from build123d import *

# Parameters (mm, degrees)
CUT_EXTRUDE1_DEPTH = 30
SKETCH3_R          = 10
CUT_EXTRUDE2_DEPTH = 30
CUT_EXTRUDE3_DEPTH = 31.3


with BuildPart() as part:
    # Sketch1 → Revolve1 (revolve)
    with BuildSketch(Plane(origin=(0, 0, 0), x_dir=(0, 0, -1), z_dir=(1, 0, 0)), mode=Mode.PRIVATE) as revolve1_sk:
        with BuildLine():
            Line((0, 20.5), (0, 15.75))
            Line((0, 15.75), (9.09326674, 0))
            Line((9.09326674, 0), (66.830344885, 0))
            Line((66.830344885, 0), (77.8, 19))
            Line((77.8, 19), (77.8, 23))
            Line((77.8, 23), (67.8, 23))
            ThreePointArc((67.8, 23), (64.1, 21.2), (60.4, 23))
            Line((60.4, 23), (38.5, 23))
            Line((38.5, 23), (36, 20.5))
            Line((36, 20.5), (0, 20.5))
        make_face()
    revolve(revolve1_sk.sketch.rotate(Axis((0, 0, 0), (0, 0, 1)), 90), axis=Axis((0, 0, 0), (0, 0, 1)))

    # Sketch2 → Cut-Extrude1 (cut)
    with BuildSketch(Plane.XY):
        with BuildLine():
            Line((-10.66, 8.821522369), (-10.66, -8.821522369))
            ThreePointArc((-10.66, -8.821522369), (-10.66, -10.66), (-8.821522369, -10.66))
            Line((-8.821522369, -10.66), (8.821522369, -10.66))
            ThreePointArc((8.821522369, -10.66), (10.66, -10.66), (10.66, -8.821522369))
            Line((10.66, -8.821522369), (10.66, 8.821522369))
            ThreePointArc((10.66, 8.821522369), (10.66, 10.66), (8.821522369, 10.66))
            Line((8.821522369, 10.66), (-8.821522369, 10.66))
            ThreePointArc((-8.821522369, 10.66), (-10.66, 10.66), (-10.66, 8.821522369))
        make_face()
    extrude(amount=-CUT_EXTRUDE1_DEPTH, mode=Mode.SUBTRACT)

    # Sketch3 → Cut-Extrude2 (cut)
    with BuildSketch(Plane.XY.offset(-30)):
        Circle(SKETCH3_R)
    extrude(amount=-CUT_EXTRUDE2_DEPTH, mode=Mode.SUBTRACT)

    # Sketch4 → Cut-Extrude3 (cut)
    with BuildSketch(Plane(origin=(0, 0, -77.8), x_dir=(-1, 0, 0), z_dir=(0, 0, -1))):
        with BuildLine():
            Line((-12.85, -9.668019485), (-12.85, 9.668019485))
            ThreePointArc((-12.85, 9.668019485), (-12.85, 12.85), (-9.668019485, 12.85))
            Line((-9.668019485, 12.85), (9.668019485, 12.85))
            ThreePointArc((9.668019485, 12.85), (12.85, 12.85), (12.85, 9.668019485))
            Line((12.85, 9.668019485), (12.85, -9.668019485))
            ThreePointArc((12.85, -9.668019485), (12.85, -12.85), (9.668019485, -12.85))
            Line((9.668019485, -12.85), (-9.668019485, -12.85))
            ThreePointArc((-9.668019485, -12.85), (-12.85, -12.85), (-12.85, -9.668019485))
        make_face()
    extrude(amount=-CUT_EXTRUDE3_DEPTH, mode=Mode.SUBTRACT)


solid = part.part
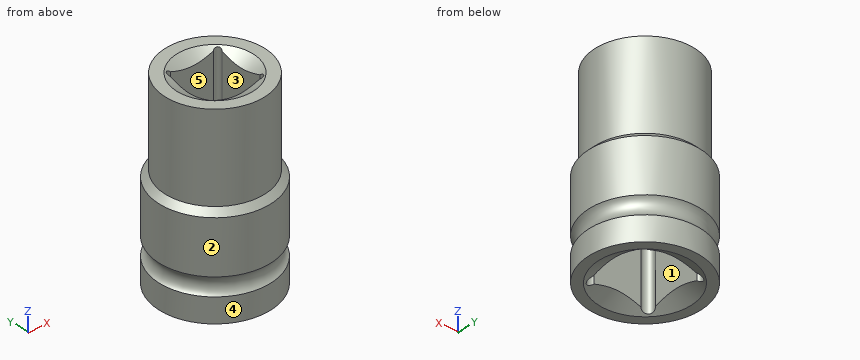
Source: CAD feature listing. Evaluate the final solid. Frame: model axes, mm. Face numbers are marked on the shaded views. A direction names the side the tool comes from. Give positions to 0.01 mm unless a question says otherwise; leave off trailing zeros. Write each loop counter-clockwise with the first axis right and the second up, starting at its lowest first coordinate (ties: lowest second). Pieces come first, ordered by that corner, then holes. Notation, with made-up numbers: M -28.75,-17 L -20.75,-17 A10 cw -20.75,2 Z; hole C -33,-15.75 d11. An arc over 180 degrees is marked long. Answer as a JSON object with one key per item and string values.
Q1. Ray query, line 1 along Y through (x, z) = (0, -41); line 2 along Y through (x, z) = (0, -35); line 3 along X through (y, z) = (-13, -50). Return the intervals inside material, ascending.
Geometry check:
{"line 1": "y = -23 to -10, 10 to 23", "line 2": "y = -20.5 to -10, 10 to 20.5", "line 3": "x = -18.97 to -12.68, -9.83 to 9.83, 12.68 to 18.97"}
Q2. Mould query, pull axis Y, two halves, no side actions, for the marked faces 4 and 5. Classes: +Y half, -Y half, draft (parallel to the pull), parting line (faces both ways), or undercut.
Geometry check:
{"face 4": "parting line", "face 5": "undercut"}
Q3. Cut plane A-A, the plane x = 0. Return the cut outline in (y, z), then the cut area to 3 significant figures.
Geometry check:
{"outline": "M -23,-77.8 L -19,-77.8 L -12.85,-74.25 L -12.85,-46.5 L -10,-46.5 L -10,-30 L -10.66,-30 L -10.66,-2.94 L -15.75,0 L -20.5,0 L -20.5,-36 L -23,-38.5 L -23,-60.4 A4.7 cw -23,-67.8 Z; M 10,-46.5 L 12.85,-46.5 L 12.85,-74.25 L 19,-77.8 L 23,-77.8 L 23,-67.8 A4.7 cw 23,-60.4 L 23,-38.5 L 20.5,-36 L 20.5,0 L 15.75,0 L 10.66,-2.94 L 10.66,-30 L 10,-30 Z", "area": "1,560 mm^2"}
Q4. Contact query for flat-ended pins moving along their axis: P1, Ø9.5, axis at x = -3.5, z = -63, coming from the +Y side; P2, Ø5, axis at x = -5, z = -25, coming from the +Y side; P3, Ø10, axis at x = 1, z = -23.5, coming from the -Y side. Output: stop coordinate, or through.
Geometry check:
{"P1": "stops at y = 23", "P2": "stops at y = 20.35", "P3": "stops at y = -20.5"}
Q5. Cut plane C-C, the plane z = -47.5. Return the cut outline in (x, y).
Geometry check:
{"outline": "C 0,0 d46; hole M -12.85,-9.67 A2.25 ccw -9.67,-12.85 L 9.67,-12.85 A2.25 ccw 12.85,-9.67 L 12.85,9.67 A2.25 ccw 9.67,12.85 L -9.67,12.85 A2.25 ccw -12.85,9.67 Z"}
Q6. Cut plane D-D, the plane z = -37. Return the cut outline in (x, y).
Geometry check:
{"outline": "C 0,0 d43; hole C 0,0 d20"}
Q7. Access query for the marked faces 1, 2 and 3. Directions: +Z, -Z, +X, -X, +Y, -Y. A direction counts if a zero-diameter tool reaches every point of the face in a straight line with its end or side. Return the directions, or none.
Geometry check:
{"face 1": "-Z", "face 2": "+Z, -Z", "face 3": "+Z"}
